CAD build for the part. Positions are in the model's coordinates, mm. Face numbers are marked on the shaded views. A direction names the side the tool comes from. Coordinates: 2 decimals unless noted, no trailing zeros. Order: outer loops, then holes, each group sorted by start corner. A loop starts at its lowest first (then second) coordinate and runs counter-clockwise, first axis right, second up.
from build123d import *

# Parameters (mm, degrees)
BOSS_EXTRUDE1_DEPTH = 5.3975
FILLET1_R           = 2.54
CUT_EXTRUDE1_DEPTH  = 10.795


with BuildPart() as part:
    # Sketch1 → Boss-Extrude1 (new, symmetric)
    with BuildSketch(Plane.XY):
        Polygon((-8.225424052, -3.67171889), (0.622258282, -36.69171889), (2.857419556, -36.69171889), (-3.632754155, -12.470060853), (4.474575948, -12.470060853), (4.474575948, -2.874424181), (-5.24987969, -2.874424181), align=None)
    extrude(amount=BOSS_EXTRUDE1_DEPTH, both=True)

    # Fillet1
    fillet1_edges = [part.edges().sort_by_distance(p)[0] for p in [
        (-3.632754155, -12.470060853, 0),
    ]]
    fillet(fillet1_edges, radius=FILLET1_R)

    # Sketch2 → Cut-Extrude1 (cut)
    with BuildSketch(Plane(origin=(-6.506920982, -1.743524222, 0), x_dir=(0, 0, -1), z_dir=(0.9659258262890691, 0.2588190451025181, 0))):
        with BuildLine():
            Line((-5.3975, -30.783533487), (-9.351765914, -30.783533487))
            Line((-9.351765914, -30.783533487), (-9.351765914, -40.742477504))
            Line((-9.351765914, -40.742477504), (7.77118576, -40.742477504))
            Line((7.77118576, -40.742477504), (7.77118576, -30.783533487))
            Line((7.77118576, -30.783533487), (5.3975, -30.783533487))
            ThreePointArc((5.3975, -30.783533487), (0, -36.181033487), (-5.3975, -30.783533487))
        make_face()
    extrude(amount=-CUT_EXTRUDE1_DEPTH, mode=Mode.SUBTRACT)


solid = part.part
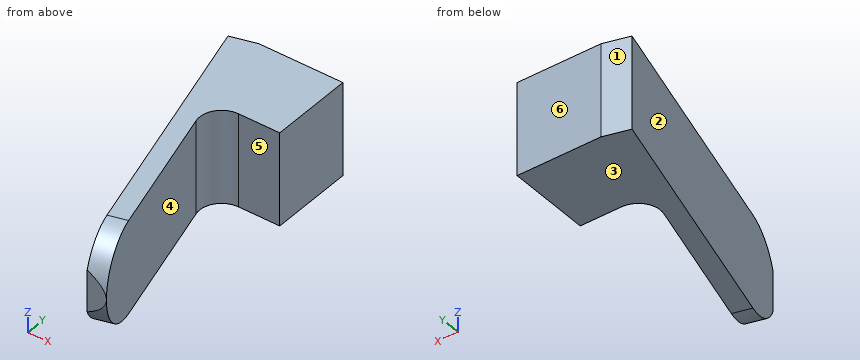
1) Slice it at C-C (z = 3.75). List the corners of the cut face in (x, y).
2) Slice it at D-D (y = -29.5). List the corners of the cut face in (x, z).
3) Two-plate mould, pull along Y, no slides. Class the marked faces 1, 2, 3 and 4: released by +Y, released by -Y, zero draft, split by the parting line, or undercut.
4) Drill centre lines: probe 1 along X at (y, z) = (-4.5, 2); probe 2 along X at (y, z) = (-31, -2); probe 3 along Z at (x, y) = (1, -32). Where is each one in solid material? Low to high.
5) Which spindle directions (+Z, -Z, +X, -X, +Y, -Y) get a long thin tool onto all of the face, cutting with end or side? Do the marked faces 5 and 6. Say none if no direction does.
6) Slice it at B-B (y = -11). List the corners of the cut face in (x, z), plus the area to 3 significant figures.
7) Pin check, flat tip, straight feed: P1, Ø1, axis at y = -16, z = 4, coming from the +X side. Stop position of the tip, or through.
8) Slice it at A-A (z = -2.75). List the corners of the cut face in (x, y), plus the area to 3 significant figures.
Worked out:
1. outline: (-8.23, -3.67) - (0.38, -35.79) - (2.47, -35.23) - (-2.78, -15.67) arc R2.54 cw to (-0.32, -12.47) - (4.47, -12.47) - (4.47, -2.87) - (-5.25, -2.87) - close
2. outline: (-1.3, -5.4) - (0.93, -5.4) - (0.93, 5.4) - (-1.3, 5.4) - close
3. face 1: released by +Y
3. face 2: released by -Y
3. face 3: zero draft
3. face 4: undercut
4. probe 1: x = -8 to 4.47
4. probe 2: x = -0.9 to 1.33
4. probe 3: z = -5.38 to 5.38
5. face 5: +Z, -Z, +X
5. face 6: +Z, -Z, +X, -X, +Y
6. outline: (-6.26, -5.4) - (4.47, -5.4) - (4.47, 5.4) - (-6.26, 5.4) - close
6. area: 116 mm2
7. P1: stops at x = -2.55
8. outline: (-8.23, -3.67) - (0.58, -36.52) - (2.66, -35.96) - (-2.78, -15.67) arc R2.54 cw to (-0.32, -12.47) - (4.47, -12.47) - (4.47, -2.87) - (-5.25, -2.87) - close
8. area: 166 mm2
